Read the model definition and answer for the solid it produces. Units are mm, in the model's axes. Face numbers are marked on the shaded views. A direction names the side the tool comes from. Give positions to 0.01 mm unless a question says otherwise; leave off trailing zeros. Order: outer loops, then holes, each group sorted by start corner. A loop starts at its lowest first (then second) coordinate and runs counter-clockwise, first axis right, second up. Notation, with made-up numbers: M 45.25,68.25 L 99.25,68.25 A18 cw 99.25,79.25 Z; hole C -28,35.25 d5. An arc over 180 degrees is marked long. One line per item, written item: value.
from build123d import *

# Parameters (mm, degrees)
EXTRUDE_1_DEPTH     = 30
SKETCH_2_R          = 1.5
EXTRUDE_2_DEPTH     = 5
SKETCH_3_R          = 1.5
CUT_EXTRUDE_1_DEPTH = 5


with BuildPart() as part:
    # 草圖1 → 填料-伸長1 (new body)
    with BuildSketch(Plane(origin=(0, 0, 0), x_dir=(1, 0, 0), z_dir=(0, 1, 0))):
        Polygon((2.886751346, 0), (1.443375673, 2.5), (-1.443375673, 2.5), (-2.886751346, 0), (-1.443375673, -2.5), (1.443375673, -2.5), align=None)
    extrude(amount=EXTRUDE_1_DEPTH)

    # 草圖2 → 填料-伸長2 (add)
    with BuildSketch(Plane(origin=(0, 30, 0), x_dir=(1, 0, 0), z_dir=(0, 1, 0))):
        Circle(SKETCH_2_R)
    extrude(amount=EXTRUDE_2_DEPTH)

    # 草圖3 → 除料-伸長1 (cut)
    with BuildSketch(Plane.XZ):
        Circle(SKETCH_3_R)
    extrude(amount=-CUT_EXTRUDE_1_DEPTH, mode=Mode.SUBTRACT)


solid = part.part
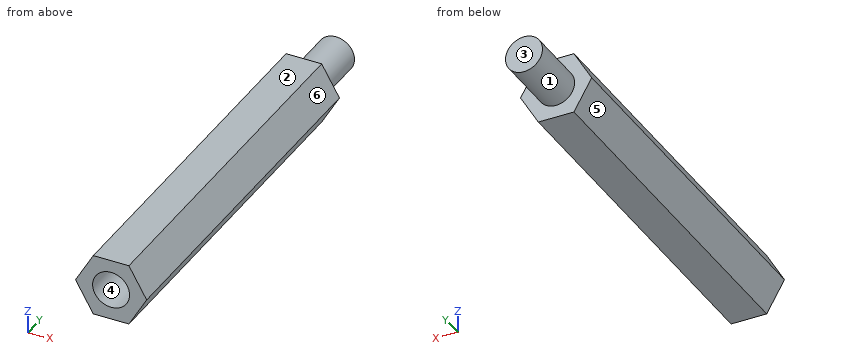
1) Find section D-D, the plane y = 32. Write down the section's boundary in (x, z), plus the area to 3 significant figures.
Reported:
outline: C 0,0 d3
area: 7.07 mm^2
2) Determine the mould class of the marked faces 3, 4, 5 and 6 for opening direction X: +X half, -X half, draft (parallel to the pull), parting line (faces both ways), or undercut.
Reported:
face 3: draft
face 4: undercut
face 5: -X half
face 6: +X half
3) Find section B-B, the plane x = 0. Write down the section's boundary in (y, z).
Reported:
outline: M 0,-2.5 L 30,-2.5 L 30,-1.5 L 35,-1.5 L 35,1.5 L 30,1.5 L 30,2.5 L 0,2.5 L 0,1.5 L 5,1.5 L 5,-1.5 L 0,-1.5 Z
4) Which of the six approach directions +Z, -Z, +X, -X, +Y, -Y give full straight-line access (tool end or side, diameter ignored) to the marked faces 1 and 2?
Reported:
face 1: +Y
face 2: +Z, +X, -X, +Y, -Y
5) Consider probe 1 along Z at (x, y) = (0, 1.7); probe 2 along Y at (x, z) = (-0.45, 0.2); probe 3 along Y at (x, z) = (-0.7, 2.2). Determine where each line is inside the solid, lowest interval first.
Reported:
probe 1: z = -2.5 to -1.5, 1.5 to 2.5
probe 2: y = 5 to 35
probe 3: y = 0 to 30
6) Find section C-C, the plane z = -0.6. Write down the section's boundary in (x, y), plus the area to 3 significant figures.
Reported:
outline: M -2.54,0 L -1.37,0 L -1.37,5 L 1.37,5 L 1.37,0 L 2.54,0 L 2.54,30 L 1.37,30 L 1.37,35 L -1.37,35 L -1.37,30 L -2.54,30 Z
area: 152 mm^2
7) Find section A-A, the plane y = 19. Write down the section's boundary in (x, z).
Reported:
outline: M -2.89,0 L -1.44,-2.5 L 1.44,-2.5 L 2.89,0 L 1.44,2.5 L -1.44,2.5 Z
8) Each of these flat-tipped pins is pushed along its axis until it touches: pin 1 Ø1 at (x, y) = (-2, 14.5) entering from +Z; pin 2 Ø3 at (y, z) = (23.5, -0.5) entering from +X; pin 3 Ø0.9 at (x, z) = (0, 0.5) entering from -Y. Where does it stop, or does it pass through?
Reported:
pin 1: stops at z = 2.4
pin 2: stops at x = 2.89
pin 3: stops at y = 5
